Autodesk Fusion 360 part; units mm, degrees
sketch "Sketch1" plane through (0, 0, 0) normal (0, 1, 0) x (1, 0, 0)
  line L0 (-60, -10) -> (60, -10)
  line L1 (60, -10) -> (60, 10)
  line L2 (60, 10) -> (-60, 10)
  line L3 (-60, 10) -> (-60, -10)
  line L4 (-60, -10) -> (60, 10) construction
  line L5 (60, -10) -> (-60, 10) construction
  line L6 (-60, -10) -> (-60, -20)
  line L7 (-40, -40) -> (40, -40)
  line L8 (60, -20) -> (60, -10)
  line L9 (39.2131, -14.2951) -> (-40, -14.2951)
  arc A0 (-40, -14.2951) -> (-40, -25.7049) centre (-40, -20) ccw
  line L10 (-40, -25.7049) -> (39.2131, -25.7049)
  arc A1 (39.2131, -25.7049) -> (39.2131, -14.2951) centre (39.2131, -20) ccw
  line L11 (39.2131, -20) -> (-40, -20) construction
  arc A2 (-60, -20) -> (-40, -40) centre (-40, -20) ccw
  arc A3 (40, -40) -> (60, -20) centre (40, -20) ccw
  point P0 (-60, -40)
  point P1 (60, -40)
  point P2 (-0.3934, -20)
  dimension "d1" = 20
  dimension "d2" = 120
  dimension "d3" = 30
  dimension "d4" = 120
  dimension "d5" = 20
  dimension "d6" = 20
  dimension "d7" = 30
extrude "Extrude1" add sketch "Sketch1" along normal blind 20
sketch "Sketch2" plane through (-60, 0, 0) normal (-1, 0, 0) x (0, -1, 0)
  line L0 (0, -10) -> (0, 20)
  line L1 (0, 20) -> (-20, 20)
  line L2 (-20, 20) -> (-20, -10)
  line L3 (-20, -10) -> (0, -10)
  line L4 (0, -10) -> (80, -10)
  line L5 (80, -10) -> (80, 10)
  line L6 (80, 10) -> (0, 10)
  line L7 (0, 10) -> (0, -10)
  dimension "d10" = 80
  dimension "d11" = 20
extrude "Extrude2" add sketch "Sketch2" against normal blind 120 contours L0 L4 L5 L6 L7
fillet "Fillet1" radius 30 2 edges at (-60, -80, 0) (60, -80, 0)
sketch "Sketch3" plane through (0, 0, 10) normal (0, 0, 1) x (-1, 0, 0)
  arc A0 (-30, 80) -> (-60, 50) centre (-30, 50) ccw
  line L0 (-60, 50) -> (-60, 0)
  line L1 (-60, 0) -> (60, 0)
  line L2 (60, 0) -> (60, 50)
  arc A1 (60, 50) -> (30, 80) centre (30, 50) ccw
  line L3 (30, 80) -> (-30, 80)
  line L4 (-30, 41.9438) -> (30, 41.9438)
  arc A2 (30, 41.9438) -> (30, 58.0562) centre (30, 50) ccw
  line L5 (30, 58.0562) -> (-30, 58.0562)
  arc A3 (-30, 58.0562) -> (-30, 41.9438) centre (-30, 50) ccw
  line L6 (-30, 50) -> (30, 50) construction
  point P0 (0, 50)
  dimension "d16" = 60
  dimension "d18" = 30
extrude "Extrude3" cut sketch "Sketch3" against normal blind 58.307 contours L4 A2 L5 A3
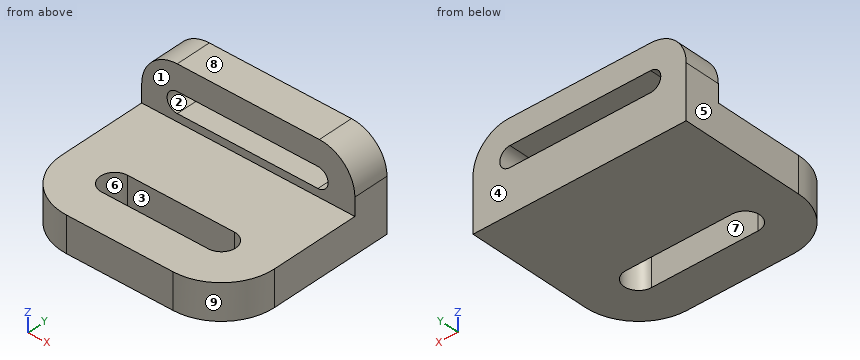
Build history of the part. All positions in model axes, mm. Face numbers are marked on the shaded views. A direction names the side the tool comes from. Coordinates: 2 decimals unless noted, no trailing zeros. Order: outer loops, then holes, each group sorted by start corner. A loop starts at its lowest first (then second) coordinate and runs counter-clockwise, first axis right, second up. Notation, with made-up numbers: (85, 28.25) - (100, 28.25) arc R31 cw to (100, 53.25) - close; hole circle Ø11 at (62, -10). An arc over 180 degrees is marked (long way). Write each question's results on one line, items separated by ' | '. Start each with the question number.
Item 1: Band-saw the part on C-C on y = 9. Write the cut outline in (x, z).
Item 2: Flat gauge pins, fed straight in: pin 1 (1.5 mm diameter, centred on x = 3, y = -65.5, fed in from +Z); pin 2 (9 mm diameter, centred on x = -4.5, z = 23.5, fed in from -Y). Where does each tip first touch, or does it go through?
Item 3: Band-saw the part on D-D on z = 18. Write the cut outline in (x, y), and give its area (3 significant figures).
Item 4: Mould opens along Y. For the marked faces 6, 7, 8 and 9 say: released by +Y, released by -Y, zero draft, split by the parting line, or undercut.
Item 5: Wall check: probe 1 along Y at (x, z) = (-18, 9); probe 2 along Z at (x, y) = (-8.5, 10.5); probe 3 along Y at (x, z) = (24.5, 29). Give the ranges that are in metal, low to high. Write a range as [from, to].
Item 6: Tool access for the marked faces 1, 2, 3, 4 and 5: list every direction of +Z, -Z, +X, -X, +Y, -Y with a clear straight run to the whole face (end or side of a thin tool).
Item 7: Band-saw the part on B-B on z = 3.5. Write the cut outline in (x, y).
Item 8: Band-saw the part on A-A on x = -5. Write the cut outline in (y, z), and give its area (3 significant figures).
Numbers:
1) outline: (-60, -10) - (60, -10) - (60, 20) arc R20 ccw to (40, 40) - (-40, 40) arc R20 ccw to (-60, 20) - close; hole (-40, 14.3) - (39.21, 14.3) arc R5.7 ccw to (39.21, 25.7) - (-40, 25.7) arc R5.7 ccw to start
2) pin 1: z = 10 | pin 2: y = 0
3) outline: (-60, 0) - (-45.34, 0) - (-45.34, 20) - (-60, 20) - close; (44.56, 0) - (60, 0) - (60, 20) - (44.56, 20) - close | area: 602 mm^2
4) face 6: undercut | face 7: undercut | face 8: zero draft | face 9: released by -Y
5) probe 1: [-80, -58.06], [-41.94, 20] | probe 2: [-10, 14.3], [25.7, 40] | probe 3: [0, 20]
6) face 1: +Z, +X, -X, -Y | face 2: +Y, -Y | face 3: +Z, -Z | face 4: +Z, -Z, +X, -X, +Y | face 5: +Z, -Z, -X, +Y, -Y
7) outline: (-60, -50) arc R30 ccw to (-30, -80) - (30, -80) arc R30 ccw to (60, -50) - (60, 20) - (-60, 20) - close; hole (-30, -58.06) - (30, -58.06) arc R8.06 ccw to (30, -41.94) - (-30, -41.94) arc R8.06 ccw to start
8) outline: (-80, -10) - (-58.06, -10) - (-58.06, 10) - (-80, 10) - close; (-41.94, -10) - (20, -10) - (20, 14.3) - (0, 14.3) - (0, 10) - (-41.94, 10) - close; (0, 25.7) - (20, 25.7) - (20, 40) - (0, 40) - close | area: 2,050 mm^2
